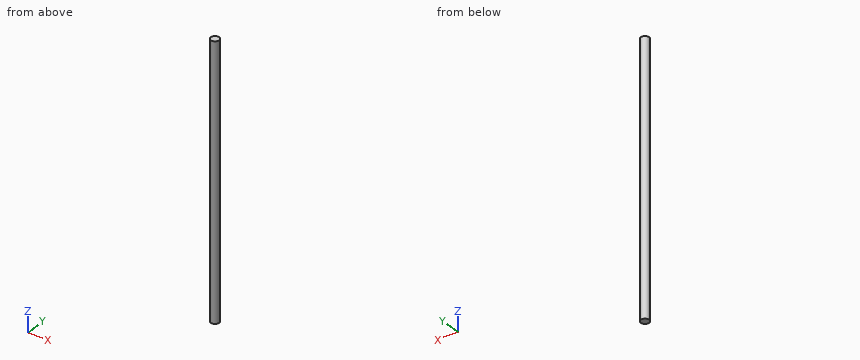
from build123d import *

# Parameters (mm, degrees)
F0_R     = 9.422662
F1_DEPTH = 254
F2_DEPTH = 609.6
F3_DEPTH = 609.6


with BuildPart() as f1:
    # F0 (on Top) → F1 (new body)
    with BuildSketch(Plane.XY):
        Circle(F0_R)
    extrude(amount=F1_DEPTH)

    # F0 (on Top) → F2 (join)
    with BuildSketch(Plane.XY):
        Circle(F0_R)
    extrude(amount=F2_DEPTH)

    # F0 (on Top) → F3 (join)
    with BuildSketch(Plane.XY):
        Circle(F0_R)
    extrude(amount=F3_DEPTH)


solid = f1.part
For this review, take the finished solid that the model builds, in its own axes (mm). Round coordinates to 2 decimals unless told otherwise and drop trailing zeros. Order: outer loops, then holes, each group sorted by start corner. A loop starts at its lowest first (then second) coordinate and runs counter-clockwise, first axis right, second up. Notation, with made-up numbers: M 85.5,51 L 117.5,51 A13 cw 117.5,67 Z; hole C 10.5,-15 d10. An arc over 180 degrees is marked long. Write each question's results on one line, items separated by ' | '. Start each with the question number.
1. Add section B-B (y = 4.25). State the section outline as (x, z) points.
2. Add section C-C (x = 5). State the section outline as (y, z) points, then the cut area to 3 significant figures.
3. Clearance check with flat-ended pins moving along their axes: pin 1 Ø6 at (x, z) = (7.5, 154) entering from -Y; pin 2 Ø1.5 at (y, z) = (-1.5, 115) entering from -X. State where each tip first meets the part, or that it passes through.
4. Add section A-A (z = 434). State the section outline as (x, y) points.
5. To check wall thickness, follow L1, parallel to X at y = -1, z = 321; L2, parallel to Y at x = -0.75, z = 585; L3, parallel to X at y = 1.5, z = 534.5. State the ranges of each line that lie inside material, in increasing order. Write a range as [from, to].
Output values:
1) outline: M -8.41,0 L 8.41,0 L 8.41,609.6 L -8.41,609.6 Z
2) outline: M -7.99,0 L 7.99,0 L 7.99,609.6 L -7.99,609.6 Z | area: 9,740 mm^2
3) pin 1: y = -8.28 | pin 2: x = -9.39
4) outline: C 0,0 d18.85
5) L1: [-9.37, 9.37] | L2: [-9.39, 9.39] | L3: [-9.3, 9.3]
